from build123d import *

# Parameters (mm, degrees)
F0_W     = 38.1
F0_H     = 76.2
F1_DEPTH = 76.2
F2_R     = 7.9375
F3_DEPTH = 59.944
F4_W     = 38.1
F4_H     = 25.4
F5_DEPTH = 19.05
F6_R     = 25.4


with BuildPart() as f1:
    # F0 (on Top) → F1 (new body)
    with BuildSketch(Plane.XY):
        with Locations((19.05, -38.1)):
            Rectangle(F0_W, F0_H)
    extrude(amount=F1_DEPTH)

    # F2 (on face) → F3 (cut)
    with BuildSketch(Plane(origin=(0, 0, 0), x_dir=(0, -1, 0), z_dir=(-1, 0, 0))):
        with Locations((38.1, 38.1)):
            Circle(F2_R)
    extrude(amount=-F3_DEPTH, mode=Mode.SUBTRACT)

    # F4 (on face) → F5 (join)
    with BuildSketch(Plane.XY.offset(76.2)):
        with Locations((19.05, -12.7)):
            Rectangle(F4_W, F4_H)
        with Locations((19.05, -63.5)):
            Rectangle(F4_W, F4_H)
    extrude(amount=F5_DEPTH)

    # F6
    f6_edges = [f1.edges().sort_by_distance(p)[0] for p in [
        (19.05, 0, 0),
        (19.05, -76.2, 0),
    ]]
    fillet(f6_edges, radius=F6_R)


solid = f1.part
Verification items for the finished model (mm, model axes). A direction names the side the tool comes from. Give positions to 0.01 mm unless a question says otherwise; leave off trailing zeros. Order: outer loops, then holes, each group sorted by start corner. A loop starts at its lowest first (then second) coordinate and runs counter-clockwise, first axis right, second up. Notation, with made-up numbers: (17.25, 44) -> (23.25, 44) arc R12 ccw to (23.25, 58) -> close; hole circle Ø3 at (-8, 70). An arc over 180 degrees is marked (long way). Answer as CSV lines item,"result".
Q1. Scan lines: probe 1 along Z at (x, y) = (18, -38); probe 2 along Y at (x, z) = (3, 88); probe 3 along Z at (x, y) = (14.5, -29). Record each from-to range of solid material in increasing order.
Solutions:
probe 1,"z = 0 to 30.16, 46.04 to 76.2"
probe 2,"y = -76.2 to -50.8, -25.4 to 0"
probe 3,"z = 0 to 76.2"
Q2. Depth check by flat-ended pin: pin 1 (2 mm diameter, centred on y = -9, z = 32.5, fed in from -X); pin 2 (7.5 mm diameter, centred on x = 22.5, y = -39, fed in from +Z). Enter the tip coordinate at first touch or a pass-through.
Solutions:
pin 1,"stops at x = 0"
pin 2,"stops at z = 76.2"
Q3. Access from +Z, -Z, +X, -X, +Y, -Y to the whole of each face (thin tool, end or side, straight path). Record for faces 1 (the flat face through (0, -39, 47)), 2 (the flat face through (19, -50.8, 86)).
Solutions:
face 1,"+Z, -Z, -X, +Y, -Y"
face 2,"+Z, +X, -X"
Q4. Sectioned sample at B-B on z = 84.5. Record the cut outline in (x, y), plus the area to 3 significant figures.
Solutions:
outline,"(0, -76.2) -> (38.1, -76.2) -> (38.1, -50.8) -> (0, -50.8) -> close; (0, -25.4) -> (38.1, -25.4) -> (38.1, 0) -> (0, 0) -> close"
area,"1,940 mm²"
Q5. Sectioned sample at D-D on z = 10.5. Record the cut outline in (x, y), plus the area to 3 significant figures.
Solutions:
outline,"(0, -71.37) -> (38.1, -71.37) -> (38.1, -4.83) -> (0, -4.83) -> close"
area,"2,540 mm²"
Q6. Release check for a two-part mould opening along Y. For faces 3 (the cylindrical face through (19.32, -68.96, 7.64)), 4 (the flat face through (19, -13, 95.25)), 5 (the flat face through (19, -25.4, 86)), 6 (the flat face through (19, 0, 60)) record: +Y half, -Y half, draft (parallel to the pull), parting line (faces both ways), or undercut.
Solutions:
face 3,"-Y half"
face 4,"draft"
face 5,"undercut"
face 6,"+Y half"
Q7. Sectioned sample at A-A on y = -38.1. Record the cut outline in (x, z).
Solutions:
outline,"(0, 0) -> (38.1, 0) -> (38.1, 30.16) -> (0, 30.16) -> close; (0, 46.04) -> (38.1, 46.04) -> (38.1, 76.2) -> (0, 76.2) -> close"
